Autodesk Inventor part; units mm, degrees
ref_plane "Work Plane1" through (12.7, 0, 0) normal (1, 0, 0) x (0, 1, 0)
ref_plane "XZ Plane" through (0, 0, 0) normal (0, 1, 0) x (-1, 0, 0)
ref_plane "XY Plane" through (0, 0, 0) normal (0, 0, 1) x (1, 0, 0)
sketch "Sketch1" plane through (0, 0, 0) normal (1, 0, 0) x (0, 1, 0)
  circle A0 centre (0, 0) radius 1.75
  arc A1 (0, 4) -> (0, -4) centre (0, 0) ccw
  line L0 (0, 0) -> (15.55, 0) construction
  line L1 (15.55, -4) -> (15.55, -6) construction
  line L2 (15.55, 0) -> (33.1, 0) construction
  arc A2 (33.1, -4) -> (33.1, 4) centre (33.1, 0) ccw
  line L3 (0, 4) -> (33.1, 4)
  arc A3 (10.9674, -4) -> (20.1326, -4) centre (15.55, -6) ccw
  circle A4 centre (15.55, -6) radius 1.75
  line L4 (0, -4) -> (10.9674, -4)
  line L5 (20.1326, -4) -> (33.1, -4)
  dimension "d0" = 3.5
  dimension "d1" = 8
  dimension "d2" = 15.55
  dimension "d4" = 17.55
  dimension "d5" = 8
  dimension "d6" = 10
  dimension "d7" = 10
  dimension "d9" = 3.5
  dimension "d37" = 15.55
extrude "Extrusion1" add sketch "Sketch1" along normal blind 6.8
sketch "Sketch2" plane through (6.8, 0, 0) normal (1, 0, 0) x (0, 0, -1)
  line L0 (0, 15.55) -> (6, 15.55) construction
  arc A0 (4, 22.7784) -> (4, 8.3216) centre (6, 15.55) ccw
  arc A1 (-4, 0) -> (4, 0) centre (0, 0) ccw construction
  line L1 (4, 0) -> (4, 8.3216) construction
  arc A2 (4, 33.1) -> (-4, 33.1) centre (0, 33.1) ccw construction
  line L2 (4, 22.7784) -> (4, 33.1) construction
  circle A3 centre (0, 0) radius 1.75
  arc A4 (-4, 0) -> (4, 0) centre (0, 0) ccw
  arc A5 (4, 33.1) -> (-4, 33.1) centre (0, 33.1) ccw
  line L3 (-4, 33.1) -> (-4, 0)
  line L4 (4, 0) -> (4, 8.3216)
  line L5 (-4, 33.1) -> (-4, 0)
  line L6 (4, 22.7784) -> (4, 33.1)
  dimension "d12" = 15.55
  dimension "d14" = 15
  dimension "d39" = 10
extrude "Extrusion2" add sketch "Sketch2" along normal blind 6.4
ref_plane "Work Plane1" through (12.7, 0, 0) normal (1, 0, 0) x (0, 1, 0)
sketch "Sketch3" plane through (12.7, 0, 0) normal (1, 0, 0) x (0, 1, 0)
  circle A0 centre (0, 0) radius 1.75
  arc A1 (0, 4) -> (0, -4) centre (0, 0) ccw
  line L0 (0, 0) -> (15.55, 0) construction
  line L1 (15.55, -4) -> (15.55, -6) construction
  line L2 (15.55, 0) -> (33.1, 0) construction
  arc A2 (33.1, -4) -> (33.1, 4) centre (33.1, 0) ccw
  line L3 (0, 4) -> (33.1, 4)
  arc A3 (10.9674, -4) -> (20.1326, -4) centre (15.55, -6) ccw
  circle A4 centre (15.55, -6) radius 1.75
  line L4 (0, -4) -> (10.9674, -4)
  line L5 (20.1326, -4) -> (33.1, -4)
  dimension "d18" = 3.5
  dimension "d19" = 8
  dimension "d20" = 15.55
  dimension "d21" = 17.55
  dimension "d22" = 8
  dimension "d23" = 10
  dimension "d24" = 10
  dimension "d26" = 3.5
  dimension "d38" = 15.55
extrude "Extrusion3" add sketch "Sketch3" along normal blind 6.8
sketch "Sketch4" plane through (0, 0, 4) normal (0, 0, 1) x (1, 0, 0)
  arc A0 (5.4, 31.35) -> (1.9, 31.35) centre (3.65, 31.35) ccw
  arc A1 (17.6, 31.35) -> (14.1, 31.35) centre (15.85, 31.35) ccw
  line L0 (0, 33.1) -> (0, 0)
  line L1 (0, 33.1) -> (19.5, 33.1)
  line L2 (19.5, 33.1) -> (19.5, 0)
  arc A2 (14.1, 27.85) -> (17.6, 27.85) centre (15.85, 27.85) ccw
  arc A3 (1.9, 27.85) -> (5.4, 27.85) centre (3.65, 27.85) ccw
  line L3 (17.6, 31.35) -> (17.6, 27.85)
  line L4 (14.1, 31.35) -> (14.1, 27.85)
  line L5 (5.4, 31.35) -> (5.4, 27.85)
  line L6 (1.9, 27.85) -> (1.9, 31.35)
  line L7 (0, 20.1326) -> (0, 33.1)
  dimension "d29" = 3.5
  dimension "d30" = 3.5
  dimension "d31" = 3.65
  dimension "d32" = 3.65
  dimension "d47" = 3.5
  dimension "d48" = 3.5
  dimension "d49" = 3.65
  dimension "d50" = 3.65
extrude "Extrusion5" cut sketch "Sketch4" against normal blind 8
sketch "Sketch5" plane through (0, 0, 0) normal (-1, 0, 0) x (0, 0, 1)
  arc A0 (4, 33.1) -> (-4, 33.1) centre (0, 33.1) ccw
  line L0 (0, 37.1) -> (0, 27.1)
  line L1 (0, 27.1) -> (-4, 27.1)
  line L2 (-4, 20.1326) -> (-4, 33.1)
  point P0 (0, 0)
  dimension "d40" = 10
  dimension "d41" = 4
extrude "Extrusion6" cut sketch "Sketch5" against normal blind 2.15
sketch "Sketch6" plane through (19.5, 0, 0) normal (1, 0, 0) x (0, 0, -1)
  point P0 (0, 0)
sketch "Sketch7" plane through (19.5, 0, 0) normal (1, 0, 0) x (0, 0, -1)
  circle A0 centre (0, 0) radius 4
  dimension "d44" = 8
extrude "Extrusion7" cut sketch "Sketch7" against normal blind 4
sketch "Sketch8" plane through (0, 0, 0) normal (-1, 0, 0) x (0, 0, 1)
  arc A0 (-4, 20.1326) -> (-4, 10.9674) centre (-6, 15.55) ccw
  circle A1 centre (-6, 15.55) radius 4
  point P0 (0, 0)
  dimension "d51" = 8
extrude "Extrusion8" cut sketch "Sketch8" against normal blind 4
properties part number "armv2"
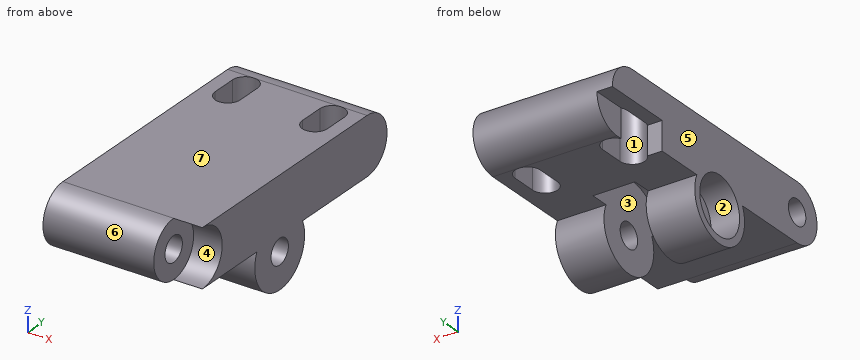
Can you work these out from the model? Positions are in its coordinate system, mm. Face numbers are marked on the shaded views. A direction names the side the tool comes from. Round coordinates to 2 decimals unless told otherwise and drop trailing zeros. Order: outer loops, then holes, each group sorted by start corner. A loop starts at its lowest first (then second) coordinate and runs counter-clockwise, first axis right, second up.
(1) If we section it at D-D (x = 11.75): Please give me the cut outline in (y, z).
Results are:
outline: (0, -4) - (8.32, -4) arc R7.5 cw to (22.78, -4) - (33.1, -4) arc R4 ccw to (33.1, 4) - (0, 4) arc R4 ccw to start; hole circle Ø3.5 at (0, 0)
(2) I'm going to push flat-ended pins straight in: pin 1 (2 mm diameter, centred on x = 8.5, z = -2, fed in from +Y); pin 2 (8 mm diameter, centred on x = 3, y = 23.5, fed in from -Z); pin 3 (1 mm diameter, centred on x = 13.5, z = -5.5, fed in from +Y); pin 4 (3 mm diameter, centred on y = 0, z = 0, fed in from -X). Where does each tip first touch, or does it pass through?
Results are:
pin 1: stops at y = 36.97
pin 2: stops at z = -9.07
pin 3: stops at y = 20.55
pin 4: passes through
(3) If we section it at C-C (z = -4.75): Please give me the cut outline in (x, y), plus the area to 3 significant figures.
Results are:
outline: (0, 10.71) - (6.8, 10.71) - (6.8, 14.33) - (4, 14.33) - (4, 11.75) - (0, 11.75) - close; (0, 19.35) - (4, 19.35) - (4, 16.77) - (6.8, 16.77) - (6.8, 20.39) - (0, 20.39) - close; (12.7, 10.71) - (19.5, 10.71) - (19.5, 14.33) - (12.7, 14.33) - close; (12.7, 16.77) - (19.5, 16.77) - (19.5, 20.39) - (12.7, 20.39) - close
area: 77.8 mm2
(4) We'd pull the mould along Z, two halves only. Please class the marked faces 4, 5, 6 and 7: +Z half, -Z half, draft (parallel to the pull), parting line (faces both ways), or undercut.
Results are:
face 4: undercut
face 5: draft
face 6: parting line
face 7: +Z half
(5) If we section it at A-A (z = -1.25): Please give me the cut outline in (x, y).
Results are:
outline: (0, -3.8) - (15.5, -3.8) - (15.5, -1.22) - (0, -1.22) - close; (0, 1.22) - (15.5, 1.22) - (15.5, 3.8) - (19.5, 3.8) - (19.5, 36.9) - (2.15, 36.9) - (2.15, 32.25) arc R1.75 cw to (5.4, 31.35) - (5.4, 27.85) arc R1.75 cw to (2.07, 27.1) - (0, 27.1) - close; hole (6.8, 9.75) - (12.7, 9.75) - (12.7, 21.35) - (6.8, 21.35) - close; hole (14.1, 27.85) arc R1.75 ccw to (17.6, 27.85) - (17.6, 31.35) arc R1.75 ccw to (14.1, 31.35) - close
(6) If we section it at B-B (x = 16.25): Please give me the cut outline in (y, z), plus the area to 3 significant figures.
Results are:
outline: (0, -4) - (10.97, -4) arc R5 ccw (long way) to (20.13, -4) - (26.15, -4) - (26.15, 4) - (0, 4) arc R4 cw to start; (33.05, -4) - (33.1, -4) arc R4 ccw to (33.1, 4) - (33.05, 4) - close; hole circle Ø3.5 at (15.55, -6)
area: 259 mm2
(7) If I drill on L1, parallel to Z at x = 8, y = 0; L2, parallel to X at y = 32.5, z = 1; L3, parallel to X at y = 16.5, z = -4, over which ranges is the centre line in solid material (lowest first)?
Results are:
L1: z = -4 to -1.75, 1.75 to 4
L2: x = 0 to 2.33, 4.97 to 14.53, 17.17 to 19.5
L3: x = 4 to 6.8, 12.7 to 19.5
(8) On a 3-axis mill with a long thin cutter (end or side, diameter ignored), from which of +Z, -Z, +X, -X, +Y, -Y can I reach the whole of each face in a straight line? I mean the marked faces 1, 2 and 3. Say none if no direction works.
Results are:
face 1: +Z, -Z
face 2: -X
face 3: -Z
